For this review, take the finished solid that the model builds, in its own axes (mm). Coordinates: 2 decimals unless noted, no trailing zeros. Write each loop counter-clockwise with the first axis right and the second up, starting at its lowest first coordinate (ties: lowest second). Pieces come first, ordered by that corner, then holes. Notation, with made-up numbers: M 2.25,31 L 16.25,31 A13 cw 16.25,49 Z; hole C 61,31.5 d5. An arc over 180 degrees is marked long. Return JSON: item names as keys, results as strings.
```python
from build123d import *

# Parameters (mm, degrees)
SKETCH020_R   = 1.5
SKETCH020_R_2 = 1
PAD034_DEPTH  = 3


with BuildPart() as part:
    # Sketch020 → Pad034 (new body)
    with BuildSketch(Plane.XY):
        Polygon((-205, -237), (22, -237), (22, -75), (35, -75), (35, 225), (-205, 225), (-205, 205), (-225, 205), (-225, -230), (-205, -230), align=None)
        with Locations((-155, 70)):
            Circle(SKETCH020_R, mode=Mode.SUBTRACT)
        with Locations((-120, 70)):
            Circle(SKETCH020_R, mode=Mode.SUBTRACT)
        with Locations((25, -40)):
            Circle(SKETCH020_R, mode=Mode.SUBTRACT)
        with Locations((25, -65)):
            Circle(SKETCH020_R, mode=Mode.SUBTRACT)
        with Locations((-120, -145)):
            Circle(SKETCH020_R, mode=Mode.SUBTRACT)
        with Locations((-155, -145)):
            Circle(SKETCH020_R, mode=Mode.SUBTRACT)
        Circle(SKETCH020_R_2, mode=Mode.SUBTRACT)
        with Locations((-20, 70)):
            Circle(SKETCH020_R, mode=Mode.SUBTRACT)
        with Locations((0, 70)):
            Circle(SKETCH020_R, mode=Mode.SUBTRACT)
        with Locations((-20, -145)):
            Circle(SKETCH020_R, mode=Mode.SUBTRACT)
        with Locations((0, -145)):
            Circle(SKETCH020_R, mode=Mode.SUBTRACT)
    extrude(amount=PAD034_DEPTH)


with BuildPart() as part_1:
    # Body035 placement: moved
    add(part.part.moved(Location((0, 0, -30))))


solid = part_1.part
```
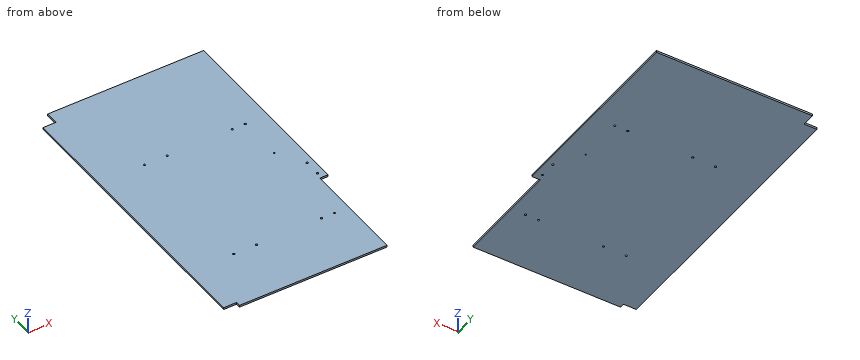
1. We need section B-B (y = -173). State the section outline as (x, z) points.
Checks:
{"outline": "M -225,-30 L 22,-30 L 22,-27 L -225,-27 Z"}
2. We need section A-A (z = -29.45). Give the number of separate pieces and of enclosed holes in the cut face, plus the area to 3 significant figures.
Checks:
{"separate pieces": "1", "enclosed holes": "11", "area": "117,000 mm2"}
3. Wall thickness on L1, parallel to Y at x = -20, z = -28.5; L2, parallel to X at y = 70, z = -28.9; L3, parallel to X at y = -145, z = -28.05: over which ranges is each line inside the solid? List them lowest first. Write a range as from..to.
Checks:
{"L1": "-237..-146.5, -143.5..68.5, 71.5..225", "L2": "-225..-156.5, -153.5..-121.5, -118.5..-21.5, -18.5..-1.5, 1.5..35", "L3": "-225..-156.5, -153.5..-121.5, -118.5..-21.5, -18.5..-1.5, 1.5..22"}
4. Clearance check with flat-ended pins moving along their axes: pin 1 Ø1.8 at (x, y) = (-120, 70) entering from -Z; pin 2 Ø1.5 at (x, z) = (26, -28.5) entering from -Y; pin 3 Ø1.5 at (y, z) = (215, -29) entering from -X; pin 4 Ø0.9 at (x, z) = (-217, -28) entering from +Y. State where each tip first meets the part, or that it passes through.
Checks:
{"pin 1": "through", "pin 2": "y = -75", "pin 3": "x = -205", "pin 4": "y = 205"}
